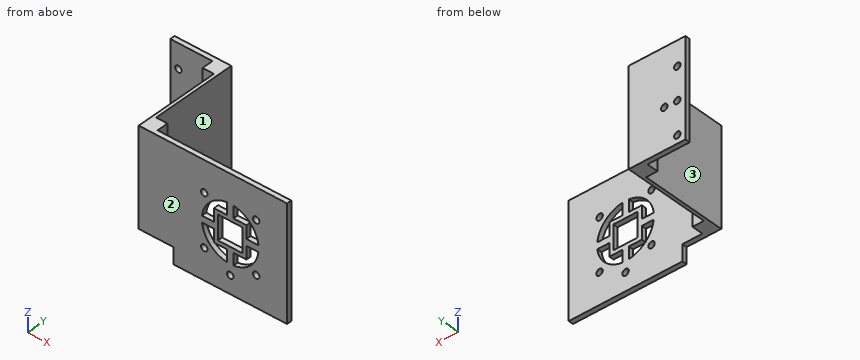
from build123d import *

# Parameters (mm, degrees)
IZIM1_W                     = 75
IZIM1_H                     = 50
Y_KSEKLIK_EKSTR_ZYON1_DEPTH = 3
IZIM8_W                     = 19.632022489
IZIM8_H                     = 50
KES_EKSTR_ZYON4_DEPTH       = 3
IZIM9_W                     = 2
IZIM9_H                     = 50
Y_KSEKLIK_EKSTR_ZYON2_DEPTH = 60
IZIM10_W                    = 35
IZIM10_H                    = 50
Y_KSEKLIK_EKSTR_ZYON3_DEPTH = 3
IZIM12_R                    = 2
KES_EKSTR_ZYON5_DEPTH       = 3
IZIM13_W                    = 20
IZIM13_H                    = 50
Y_KSEKLIK_EKSTR_ZYON4_DEPTH = 3
IZIM14_R                    = 2
KES_EKSTR_ZYON6_DEPTH       = 3
IZIM15_W                    = 15
IZIM15_H                    = 15
KES_EKSTR_ZYON7_DEPTH       = 3
KES_EKSTR_ZYON8_DEPTH       = 3
IZIM17_W                    = 5
IZIM17_H                    = 50
Y_KSEKLIK_EKSTR_ZYON5_DEPTH = 3
Y_KSEKLIK_EKSTR_ZYON6_DEPTH = 3
IZIM19_R                    = 2
KES_EKSTR_ZYON9_DEPTH       = 3
IZIM20_W                    = 7
IZIM20_H                    = 7
Y_KSEKLIK_EKSTR_ZYON7_DEPTH = 50
Y_KSEKLIK_EKSTR_ZYON8_DEPTH = 10


with BuildPart() as part:
    # Çizim1 → Yükseklik-Ekstrüzyon1 (new body)
    with BuildSketch(Plane(origin=(0, 0, 0), x_dir=(1, 0, 0), z_dir=(0, 1, 0))):
        Rectangle(IZIM1_W, IZIM1_H)
    extrude(amount=Y_KSEKLIK_EKSTR_ZYON1_DEPTH)

    # Çizim8 → Kes-Ekstrüzyon4 (cut)
    with BuildSketch(Plane(origin=(0, 3, 0), x_dir=(1, 0, 0), z_dir=(0, 1, 0))):
        with Locations((-27.683988755, 0)):
            Rectangle(IZIM8_W, IZIM8_H)
    extrude(amount=-KES_EKSTR_ZYON4_DEPTH, mode=Mode.SUBTRACT)

    # Çizim9 → Yükseklik-Ekstrüzyon2 (add)
    with BuildSketch(Plane(origin=(0, 0, 0), x_dir=(1, 0, 0), z_dir=(0, 1, 0))):
        with Locations((-18.867977511, 0)):
            Rectangle(IZIM9_W, IZIM9_H)
    extrude(amount=Y_KSEKLIK_EKSTR_ZYON2_DEPTH)

    # Çizim10 → Yükseklik-Ekstrüzyon3 (add)
    with BuildSketch(Plane(origin=(0, 60, 0), x_dir=(1, 0, 0), z_dir=(0, 1, 0))):
        with Locations((-35.367977511, 0)):
            Rectangle(IZIM10_W, IZIM10_H)
    extrude(amount=Y_KSEKLIK_EKSTR_ZYON3_DEPTH)

    # Çizim12 → Kes-Ekstrüzyon5 (cut)
    with BuildSketch(Plane(origin=(0, 63, 0), x_dir=(1, 0, 0), z_dir=(0, 1, 0))):
        with Locations(Location((-39.867977511, 0, 0), (0, 0, 270))):
            Circle(IZIM12_R)
        with Locations(Location((-47.867977511, 0, 0), (0, 0, 270))):
            Circle(IZIM12_R)
        with Locations(Location((-47.867977511, 20, 0), (0, 0, 270))):
            Circle(IZIM12_R)
        with Locations(Location((-47.867977511, -20, 0), (0, 0, 270))):
            Circle(IZIM12_R)
    extrude(amount=-KES_EKSTR_ZYON5_DEPTH, mode=Mode.SUBTRACT)

    # Çizim13 → Yükseklik-Ekstrüzyon4 (add)
    with BuildSketch(Plane(origin=(0, 3, 0), x_dir=(1, 0, 0), z_dir=(0, 1, 0))):
        with Locations((47.5, 0)):
            Rectangle(IZIM13_W, IZIM13_H)
    extrude(amount=-Y_KSEKLIK_EKSTR_ZYON4_DEPTH)

    # Çizim14 → Kes-Ekstrüzyon6 (cut)
    with BuildSketch(Plane(origin=(0, 3, 0), x_dir=(1, 0, 0), z_dir=(0, 1, 0))):
        with Locations(Location((20.5, 16, 0), (0, 0, 270))):
            Circle(IZIM14_R)
        with Locations(Location((52.5, 16, 0), (0, 0, 270))):
            Circle(IZIM14_R)
        with Locations(Location((20.5, -16, 0), (0, 0, 270))):
            Circle(IZIM14_R)
        with Locations(Location((52.5, -16, 0), (0, 0, 270))):
            Circle(IZIM14_R)
    extrude(amount=-KES_EKSTR_ZYON6_DEPTH, mode=Mode.SUBTRACT)

    # Çizim15 → Kes-Ekstrüzyon7 (cut)
    with BuildSketch(Plane(origin=(0, 3, 0), x_dir=(1, 0, 0), z_dir=(0, 1, 0))):
        with Locations((36.5, 0)):
            Rectangle(IZIM15_W, IZIM15_H)
    extrude(amount=-KES_EKSTR_ZYON7_DEPTH, mode=Mode.SUBTRACT)

    # Çizim16 → Kes-Ekstrüzyon8 (cut)
    with BuildSketch(Plane(origin=(0, 3, 0), x_dir=(1, 0, 0), z_dir=(0, 1, 0))):
        with BuildLine():
            Line((46.5, 2), (53.885338651, 2))
            ThreePointArc((53.885338651, 2), (48.874368671, 12.374368671), (38.5, 17.385338651))
            Line((38.5, 17.385338651), (38.5, 10))
            Line((38.5, 10), (46.5, 10))
            Line((46.5, 10), (46.5, 2))
        make_face()
        with BuildLine():
            Line((26.5, 10), (34.5, 10))
            Line((34.5, 10), (34.5, 17.385338651))
            ThreePointArc((34.5, 17.385338651), (24.125631329, 12.374368671), (19.114661349, 2))
            Line((19.114661349, 2), (26.5, 2))
            Line((26.5, 2), (26.5, 10))
        make_face()
        with BuildLine():
            Line((26.5, -10), (34.5, -10))
            Line((34.5, -10), (34.5, -17.385338651))
            ThreePointArc((34.5, -17.385338651), (24.125631329, -12.374368671), (19.114661349, -2))
            Line((19.114661349, -2), (26.5, -2))
            Line((26.5, -2), (26.5, -10))
        make_face()
        with BuildLine():
            Line((46.5, -2), (53.885338651, -2))
            ThreePointArc((53.885338651, -2), (48.874368671, -12.374368671), (38.5, -17.385338651))
            Line((38.5, -17.385338651), (38.5, -10))
            Line((38.5, -10), (46.5, -10))
            Line((46.5, -10), (46.5, -2))
        make_face()
    extrude(amount=-KES_EKSTR_ZYON8_DEPTH, mode=Mode.SUBTRACT)

    # Çizim17 → Yükseklik-Ekstrüzyon5 (add)
    with BuildSketch(Plane(origin=(0, 3, 0), x_dir=(1, 0, 0), z_dir=(0, 1, 0))):
        with Locations((60, 0)):
            Rectangle(IZIM17_W, IZIM17_H)
    extrude(amount=-Y_KSEKLIK_EKSTR_ZYON5_DEPTH)

    # Çizim18 → Yükseklik-Ekstrüzyon6 (add)
    with BuildSketch(Plane(origin=(0, 3, 0), x_dir=(1, 0, 0), z_dir=(0, 1, 0))):
        Polygon((1.5, 25), (62.5, 25), (62.5, -25), (1.5, -25), (1.5, -35), (71.5, -35), (71.5, 35), (1.5, 35), align=None)
    extrude(amount=-Y_KSEKLIK_EKSTR_ZYON6_DEPTH)

    # Çizim19 → Kes-Ekstrüzyon9 (cut)
    with BuildSketch(Plane(origin=(0, 3, 0), x_dir=(1, 0, 0), z_dir=(0, 1, 0))):
        with Locations(Location((36.5, 24, 0), (0, 0, 270))):
            Circle(IZIM19_R)
    extrude(amount=-KES_EKSTR_ZYON9_DEPTH, mode=Mode.SUBTRACT)

    # Çizim20 → Yükseklik-Ekstrüzyon7 (add)
    with BuildSketch(Plane.XY.offset(25)):
        with Locations((-23.367977511, 56.5)):
            Rectangle(IZIM20_W, IZIM20_H)
        with Locations((-14.367977511, 6.5)):
            Rectangle(IZIM20_W, IZIM20_H)
    extrude(amount=-Y_KSEKLIK_EKSTR_ZYON7_DEPTH)

    # Çizim21 → Yükseklik-Ekstrüzyon8 (add)
    with BuildSketch(Plane.XY.offset(25)):
        Polygon((-52.867977511, 60), (-52.867977511, 63), (-17.867977511, 63), (-17.867977511, 10), (-10.867977511, 10), (-10.867977511, 3), (1.5, 3), (1.5, 0), (-19.867977511, 0), (-19.867977511, 53), (-26.867977511, 53), (-26.867977511, 60), align=None)
    extrude(amount=Y_KSEKLIK_EKSTR_ZYON8_DEPTH)


solid = part.part
Can you work these out from the model? Positions are in its coordinate system, mm. Face numbers are marked on the shaded views. A direction names the side the tool comes from. Give positions to 0.01 mm unless a question says otherwise; leave off trailing zeros. Order: outer loops, then holes, each group sorted by start corner. A loop starts at its lowest first (then second) coordinate and runs counter-clockwise, first axis right, second up. Notation, with made-up numbers: M 51.5,54 L 63.5,54 A26 cw 63.5,81 Z; hole C 25,-9 d5. An arc over 180 degrees is marked long. Use one line per item in the form item = value. Start each with the question number.
Item 1: If we section it at D-D (x = 52.5): Write out the boundary of the cut face in (y, z).
Item 2: Will these pins go through, and if not, where does the flat tip stop? pin 1 Ø8 at (y, z) = (23, -18.5) entering from -X; pin 2 Ø1.5 at (x, z) = (29.5, 4) entering from +Y; pin 3 Ø7.5 at (x, z) = (-24, 17.5) entering from -Y.
Item 3: If I drill on line 1 along X through (y, z) = (61, -20); line 2 along Y through (x, z) = (18.5, 31.5); line 3 along X through (y, z) = (48.5, 21.5), over which ranges is the centre line in solid material (lowest first)?
Item 4: For the marked faces 1, 2 and 3, which set-ups out of +Z, -Z, +X, -X, +Y, -Y let a thin tool reach every point of the face, with its end or its side?
Item 5: If we section it at C-C (z = -16): Write out the boundary of the cut face in (x, y).
Item 6: If we section it at A-A (z = 20.5): Write out the boundary of the cut face in (x, y), then the cut area to 3 significant figures.
Item 7: If we section it at B-B (x = 36.5): Write out the boundary of the cut face in (y, z), then the cut area to 3 significant figures.
Outcome:
q1.outline = M 0,-35 L 3,-35 L 3,-18 L 0,-18 Z; M 0,-14 L 3,-14 L 3,-7.09 L 0,-7.09 Z; M 0,-2 L 3,-2 L 3,2 L 0,2 Z; M 0,7.09 L 3,7.09 L 3,14 L 0,14 Z; M 0,18 L 3,18 L 3,35 L 0,35 Z
q2.pin_1 = -19.87
q2.pin_2 = 3
q2.pin_3 = 53
q3.line_1 = -52.87 to -49.87, -45.87 to -17.87
q3.line_2 = 0 to 3
q3.line_3 = -19.87 to -17.87
q4.face_1 = +Z, -Z, +X, +Y
q4.face_2 = +Z, -Z, +X, -X, -Y
q4.face_3 = +Z, -Z, -X, -Y
q5.outline = M -52.87,60 L -26.87,60 L -26.87,53 L -19.87,53 L -19.87,0 L 18.5,0 L 18.5,3 L -10.87,3 L -10.87,10 L -17.87,10 L -17.87,63 L -52.87,63 Z; M 22.5,0 L 29.41,0 L 29.41,3 L 22.5,3 Z; M 34.5,0 L 38.5,0 L 38.5,3 L 34.5,3 Z; M 43.59,0 L 50.5,0 L 50.5,3 L 43.59,3 Z; M 54.5,0 L 71.5,0 L 71.5,3 L 54.5,3 Z
q6.outline = M -52.87,60 L -49.8,60 L -49.8,63 L -52.87,63 Z; M -45.93,60 L -26.87,60 L -26.87,53 L -19.87,53 L -19.87,0 L 71.5,0 L 71.5,3 L -10.87,3 L -10.87,10 L -17.87,10 L -17.87,63 L -45.93,63 Z
q6.area = 579 mm2
q7.outline = M 0,-35 L 3,-35 L 3,-26 L 0,-26 Z; M 0,-22 L 3,-22 L 3,-7.5 L 0,-7.5 Z; M 0,7.5 L 3,7.5 L 3,35 L 0,35 Z
q7.area = 153 mm2
